Can you work these out from the drawing? Everything is in mm from the part's minimum corner. A direction names the side the tool comes from. Round coordinates to 2 decimals unless told otherwise and drop trailing zeros. Write each loop counter-clockwise with the first axis right and the second up, starting at its lowest first coordinate (ties: lowest second). Pieces come first, ordered by that corner, then holes.
Q1. We'd pull the mould along Y, two halves only. Please class the marked faces 1, 2 and 3: +Y half, -Y half, draft (parallel to the pull), parting line (faces both ways), or undercut.
Q2. If we section it at D-D (x = 2.5): Please give me the cut outline in (y, z).
Q3. I'm going to push flat-ended pins straight in: pin 1 Ø1.5 at (y, z) = (1, 16.5) entering from +X; pin 2 Ø5 at (x, z) = (4.5, 31) entering from +Y; pin 3 Ø4.5 at (x, y) = (14, 4.75) entering from -Z; pin 4 Ø1 at (y, z) = (2.5, 28.5) entering from +X. Where does each tip first touch, or does it pass through?
Q4. Please list where these lines run through material, in increasing order: line 1 along Z through (x, y) = (10.5, 2); line 2 along Y through (x, z) = (14, 28); line 3 along Y through (x, z) = (4, 23).
Q5. If we section it at B-B (x = 4.5): Please give me the cut outline in (y, z).
Q6. For the marked faces 4 and 5, which set-ups out of +Z, -Z, +X, -X, +Y, -Y let a thin tool reach every point of the face, with its end or its side?
Q7. If we section it at A-A (z = 6): Please give me the cut outline in (x, y).
Q8. If we section it at C-C (y = 6.5): Please give me the cut outline in (x, z) (1 decimal).
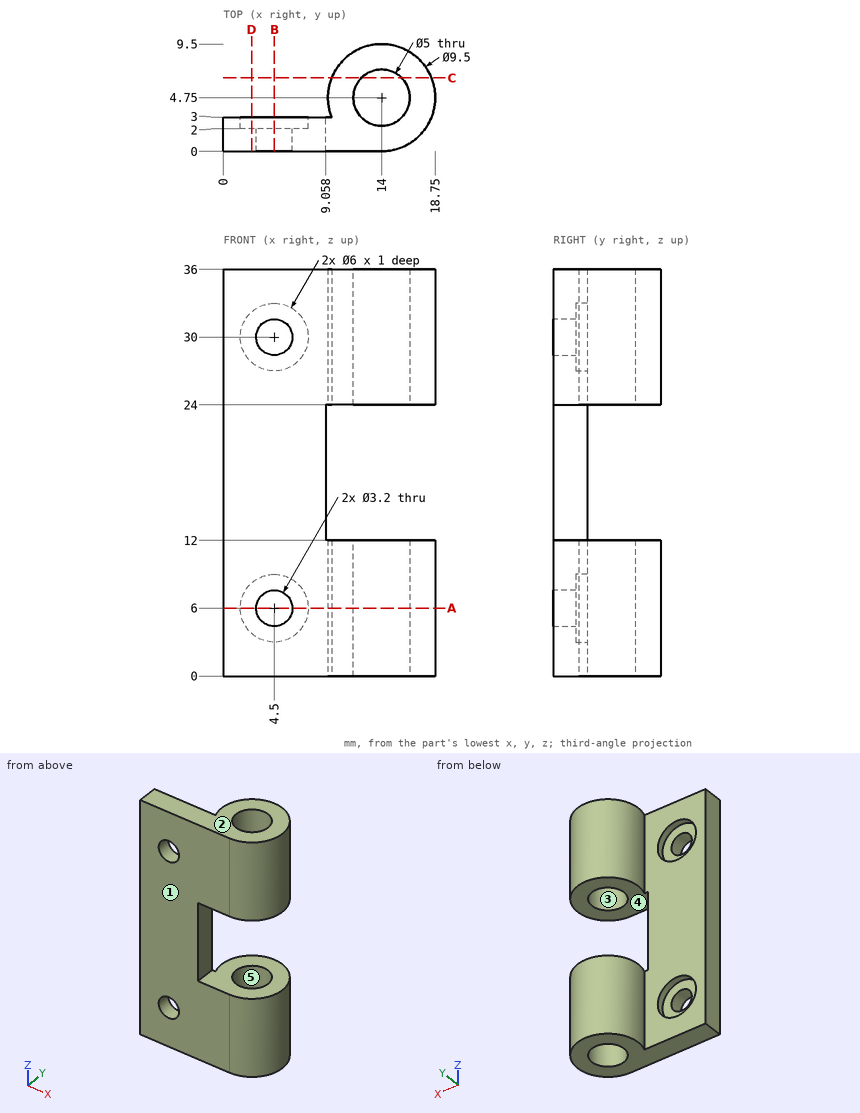
A:
1. face 1: -Y half
1. face 2: draft
1. face 3: undercut
2. outline: (0, 0) - (3, 0) - (3, 3.76) - (2, 3.76) - (2, 8.24) - (3, 8.24) - (3, 27.76) - (2, 27.76) - (2, 32.24) - (3, 32.24) - (3, 36) - (0, 36) - close
3. pin 1: stops at x = 9.06
3. pin 2: stops at y = 3
3. pin 3: passes through
3. pin 4: stops at x = 18.42
4. line 1: z = 0 to 12, 24 to 36
4. line 2: y = 0 to 2.25, 7.25 to 9.5
4. line 3: y = 0 to 3
5. outline: (0, 0) - (3, 0) - (3, 3) - (2, 3) - (2, 4.4) - (0, 4.4) - close; (0, 7.6) - (2, 7.6) - (2, 9) - (3, 9) - (3, 27) - (2, 27) - (2, 28.4) - (0, 28.4) - close; (0, 31.6) - (2, 31.6) - (2, 33) - (3, 33) - (3, 36) - (0, 36) - close
6. face 4: +X, +Y, -Y
6. face 5: +Z, -Z
7. outline: (0, 0) - (2.9, 0) - (2.9, 2) - (1.5, 2) - (1.5, 3) - (0, 3) - close; (6.1, 0) - (14, 0) arc R4.75 ccw (long way) to (9.58, 3) - (7.5, 3) - (7.5, 2) - (6.1, 2) - close; hole circle Ø5 at (14, 4.75)
8. outline: (9.6, 0) - (12.2, 0) - (12.2, 12) - (9.6, 12) - close; (9.6, 24) - (12.2, 24) - (12.2, 36) - (9.6, 36) - close; (15.8, 0) - (18.4, 0) - (18.4, 12) - (15.8, 12) - close; (15.8, 24) - (18.4, 24) - (18.4, 36) - (15.8, 36) - close
